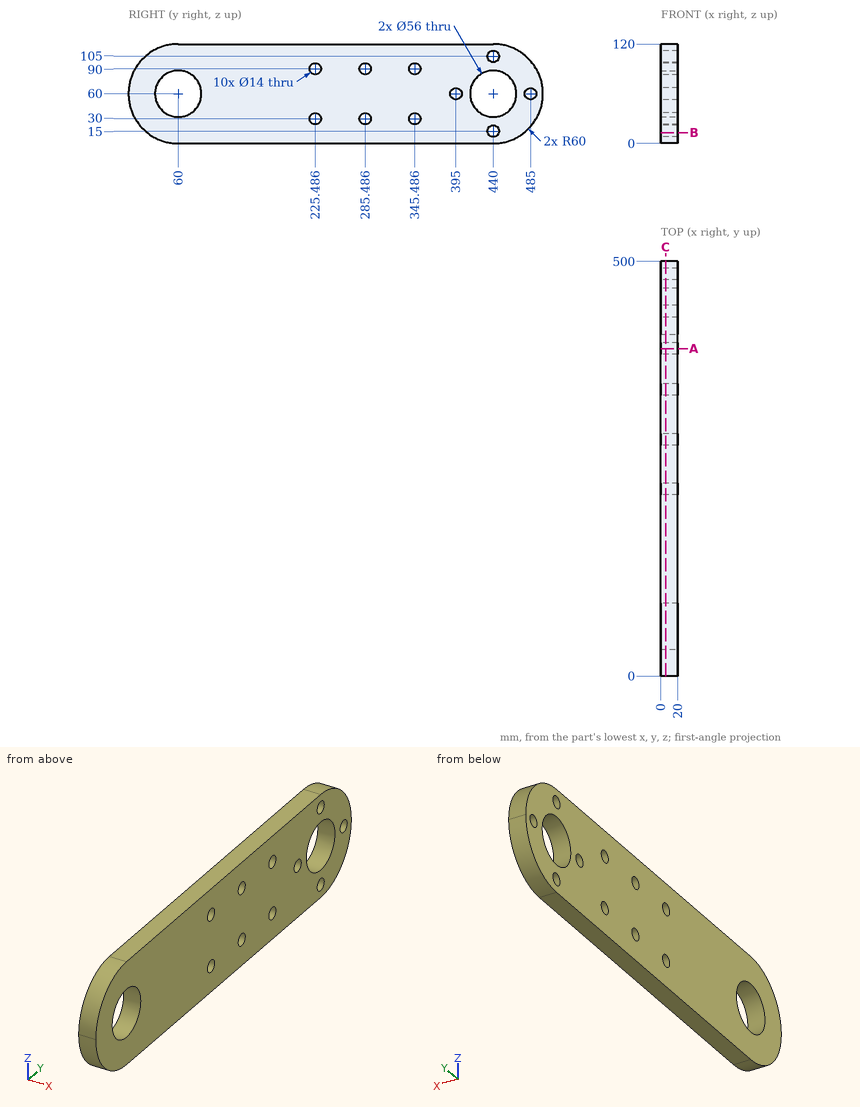
Geometry check sheet. Reference: drawing and pictorial views, mm from the part's lowest x, y, z. Coordinates: 2 decimals unless noted, no trailing zeros. Loops run counter-clockwise (first coordinate to the right, second up) from the corner with the lowest first, then second, coordinate; pieces in that order, holes last.
1) Sectioned sample at C-C (x = 5.75). Count the separate pieces of the cut face and the enclosed holes in it, and give its area (3 significant figures).
2) Material ranges on probe 1 along Y at (x, z) = (14, 90); probe 2 along Z at (x, y) = (12, 229.5) (1 decimal); probe 3 along Y at (x, z) = (1.25, 68), recorded low to high.
3) Sectioned sample at B-B (z = 13). Record the boundary of the cut face in (x, y).
4) Gauge pin test, flat ends, axial feed: pin 1 (18 mm diameter, centred on y = 285.49, z = 90, fed in from +X); pin 2 (2 mm diameter, centred on x = 16.5, z = 80.5, fed in from +Y); pin 3 (4 mm diameter, centred on x = 6, z = 26, fed in from +Y); pin 4 (1.5 mm diameter, centred on x = 2.5, z = 97, fed in from -Y). Record the tip position at first contact, or that the pin passes through.
5) Sectioned sample at A-A (y = 395). Record the boundary of the cut face in (x, z).
Check sheet entries:
1. separate pieces: 1
1. enclosed holes: 12
1. area: 50,400 mm2
2. probe 1: y = 8.04 to 218.49, 232.49 to 278.49, 292.49 to 338.49, 352.49 to 491.96
2. probe 2: z = 0 to 24.3, 35.7 to 84.3, 95.7 to 120
2. probe 3: y = 0.54 to 33.17, 86.83 to 413.17, 466.83 to 499.46
3. outline: (0, 22.7) - (20, 22.7) - (20, 433.29) - (0, 433.29) - close; (0, 446.71) - (20, 446.71) - (20, 477.3) - (0, 477.3) - close
4. pin 1: stops at x = 20
4. pin 2: stops at y = 496.74
4. pin 3: stops at y = 490.75
4. pin 4: stops at y = 12.19
5. outline: (0, 0) - (20, 0) - (20, 53) - (0, 53) - close; (0, 67) - (20, 67) - (20, 120) - (0, 120) - close
